```python
from build123d import *

# Parameters (mm, degrees)
BOSS_EXTRUDE1_DEPTH = 25.4
BOSS_EXTRUDE2_DEPTH = 6.35
SKETCH2_W           = 12.7
SKETCH2_H           = 38.1
CUT_EXTRUDE1_DEPTH  = 10.16
SKETCH3_W           = 12.7
SKETCH3_H           = 24.13
CUT_EXTRUDE2_DEPTH  = 16.24
SKETCH4_R           = 1.016
CUT_EXTRUDE3_DEPTH  = 12.7
SKETCH6_R           = 3.175
CUT_EXTRUDE4_DEPTH  = 7.35
CIRPATTERN1_COUNT   = 6


with BuildPart() as part:
    # Sketch1 → Boss-Extrude1 (new body)
    with BuildSketch(Plane(origin=(0, 0, 0), x_dir=(1, 0, 0), z_dir=(0, 1, 0))):
        Polygon((58.65878735, 0), (29.329393675, 50.8), (-29.329393675, 50.8), (-58.65878735, 0), (-29.329393675, -50.8), (29.329393675, -50.8), align=None)
    extrude(amount=BOSS_EXTRUDE1_DEPTH)

    # Sketch5 → Boss-Extrude2 (add)
    with BuildSketch(Plane.XZ):
        Polygon((87.988181024, 0), (43.994090512, 76.2), (-43.994090512, 76.2), (-87.988181024, 0), (-43.994090512, -76.2), (43.994090512, -76.2), align=None)
        Polygon((58.65878735, 0), (29.329393675, 50.8), (-29.329393675, 50.8), (-58.65878735, 0), (-29.329393675, -50.8), (29.329393675, -50.8), align=None, mode=Mode.SUBTRACT)
    extrude(amount=-BOSS_EXTRUDE2_DEPTH)

    # Sketch2 → Cut-Extrude1 (cut)
    with BuildSketch(Plane(origin=(0, 25.4, 0), x_dir=(1, 0, 0), z_dir=(0, 1, 0))):
        with Locations((0, -31.75)):
            Rectangle(SKETCH2_W, SKETCH2_H)
    cut_extrude1 = extrude(amount=-CUT_EXTRUDE1_DEPTH, mode=Mode.SUBTRACT)

    # Sketch3 → Cut-Extrude2 (cut, through all)
    with BuildSketch(Plane(origin=(0, 15.24, 0), x_dir=(1, 0, 0), z_dir=(0, 1, 0))):
        with Locations((0, -33.655)):
            Rectangle(SKETCH3_W, SKETCH3_H)
    cut_extrude2 = extrude(amount=-CUT_EXTRUDE2_DEPTH, mode=Mode.SUBTRACT)

    # Sketch4 → Cut-Extrude3 (cut)
    with BuildSketch(Plane(origin=(0, 15.24, 0), x_dir=(1, 0, 0), z_dir=(0, 1, 0))):
        with Locations((0, -19.812)):
            Circle(SKETCH4_R)
        with Locations((0, -46.99)):
            Circle(SKETCH4_R)
    cut_extrude3 = extrude(amount=-CUT_EXTRUDE3_DEPTH, mode=Mode.SUBTRACT)

    # Sketch6 → Cut-Extrude4 (cut, through all)
    with BuildSketch(Plane(origin=(0, 6.35, 0), x_dir=(1, 0, 0), z_dir=(0, 1, 0))):
        with Locations((0, -63.5)):
            Circle(SKETCH6_R)
    cut_extrude4 = extrude(amount=-CUT_EXTRUDE4_DEPTH, mode=Mode.SUBTRACT)

    # CirPattern1: Cut-Extrude1, Cut-Extrude2, Cut-Extrude3, Cut-Extrude4 ×6 about axis
    cirpattern1_axis = Axis((0, 0, 0), (0, 1, 0))
    for i in range(1, CIRPATTERN1_COUNT):
        add(cut_extrude1.rotate(cirpattern1_axis, i * 360 / CIRPATTERN1_COUNT), mode=Mode.SUBTRACT)
        add(cut_extrude2.rotate(cirpattern1_axis, i * 360 / CIRPATTERN1_COUNT), mode=Mode.SUBTRACT)
        add(cut_extrude3.rotate(cirpattern1_axis, i * 360 / CIRPATTERN1_COUNT), mode=Mode.SUBTRACT)
        add(cut_extrude4.rotate(cirpattern1_axis, i * 360 / CIRPATTERN1_COUNT), mode=Mode.SUBTRACT)


solid = part.part
```
Check sheet for the modelled part. Datum: model origin and axes. Units: mm. A direction names the side the tool comes from. Round coordinates to 2 decimals unless told otherwise and drop trailing zeros. Write each loop counter-clockwise with the first axis right and the second up, starting at its lowest first coordinate (ties: lowest second). Pieces come first, ordered by that corner, then holes. Notation, with made-up numbers: (64, 0.5) -> (82, 0.5) arc R14 cw to (82, 25.5) -> close; hole circle Ø1 at (-24.75, 55.5). An arc over 180 degrees is marked (long way). Put each result on its own line as item: value.
(1) Material ranges on line 1 (Z direction, x = 5, y = 6.25); line 2 (X direction, y = 16, z = 18); line 3 (X direction, y = 20.25, z = -3), recorded low to high.
Values found:
line 1: z = -76.2 to -45.72, -21.59 to 21.59, 45.72 to 76.2
line 2: x = -48.27 to -43.88, -18.48 to -6.35, 6.35 to 18.48, 43.88 to 48.27
line 3: x = -56.93 to -17.9, -12.93 to 12.93, 17.9 to 56.93
(2) Go/stop test with flat-tipped pins: pin 1 Ø1 at (x, y) = (-23, 21) entering from +Z; pin 2 Ø1.2 at (x, z) = (0, -19.812) entering from +Y; pin 3 Ø8.5 at (x, z) = (41.5, 26) entering from +Y. Record where each tip stops, or that it passes through.
Values found:
pin 1: stops at z = 50.8
pin 2: stops at y = 2.54
pin 3: stops at y = 15.24
(3) Tool access check on faces 1 (the face through (0, 15.24, -17)), 2 (the face through (-66.299, 3.131, -37.567)), 3 (the face through (-39.64, 7.73, 22.78)), 4 (the face through (11.043, 20.391, -6.273)). Record the directions out of +Z, -Z, +X, -X, +Y, -Y that give a thin tool (end or side, any length) a straight path to the whole face; none if there is none.
Values found:
face 1: -Z, +Y
face 2: -Z, -X, +Y, -Y
face 3: +Y, -Y
face 4: +Y
(4) Sectioned sample at C-C (z = -63.5). Enter the section's corners in (x, y) (3 decimals), plus the area to 3 significant figures.
Values found:
outline: (-51.326, 0) -> (-3.175, 0) -> (-3.175, 6.35) -> (-51.326, 6.35) -> close; (3.175, 0) -> (51.326, 0) -> (51.326, 6.35) -> (3.175, 6.35) -> close
area: 612 mm^2
(5) Mould release check, pull along X, two halves, no side actions. Record for faces 5 (the face through (-6.35, 13, -32)), 6 (the face through (0, 14, -50.8)), 7 (the face through (39.64, 7.73, -22.78)), 8 (the face through (-44.2, 13.62, 25.04)): released by +X, released by -X, zero draft, split by the parting line, or undercut.
Values found:
face 5: undercut
face 6: zero draft
face 7: undercut
face 8: released by -X
(6) Sectioned sample at D-D (x = -75.5). Enter the section's corners in (y, z).
Values found:
outline: (0, -21.63) -> (6.35, -21.63) -> (6.35, 21.63) -> (0, 21.63) -> close
(7) Sectioned sample at B-B (x = 32.5). Enter the section's corners in (y, z), plus the area to 3 significant figures.
Values found:
outline: (0, -76.2) -> (6.35, -76.2) -> (6.35, -45.31) -> (25.4, -45.31) -> (25.4, -26.1) -> (0, -26.1) -> close; (0, -11.43) -> (25.4, -11.43) -> (25.4, 11.43) -> (0, 11.43) -> close; (0, 26.1) -> (25.4, 26.1) -> (25.4, 45.31) -> (6.35, 45.31) -> (6.35, 76.2) -> (0, 76.2) -> close
area: 1,950 mm^2
